```python
from build123d import *

# Parameters (mm, degrees)
F1_DEPTH = 50.8
F2_W     = 22.225
F2_H     = 25.4
F3_DEPTH = 44.704
F4_W     = 22.225
F4_H     = 25.4
F5_DEPTH = 37.592


with BuildPart() as f1:
    # F0 (on Top) → F1 (new body)
    with BuildSketch(Plane.XY):
        Polygon((60.325, 31.75), (-60.325, 31.75), (-60.325, -3.175), (-10.831648, -31.75), (10.831648, -31.75), (60.325, -3.175), align=None)
    extrude(amount=F1_DEPTH)

    # F2 (on Front) → F3 (cut, symmetric)
    with BuildSketch(Plane.XZ):
        with Locations((-49.2125, 38.1)):
            Rectangle(F2_W, F2_H)
    extrude(amount=F3_DEPTH, both=True, mode=Mode.SUBTRACT)

    # F4 (on Front) → F5 (cut, symmetric)
    with BuildSketch(Plane.XZ):
        with Locations((49.2125, 38.1)):
            Rectangle(F4_W, F4_H)
    extrude(amount=F5_DEPTH, both=True, mode=Mode.SUBTRACT)


solid = f1.part
```
The listing builds one solid part. Answer for the finished solid, in the listing's coordinates (mm). A direction names the side the tool comes from. Round coordinates to 2 decimals unless told otherwise and drop trailing zeros. Loops run counter-clockwise (first coordinate to the right, second up) from the corner with the lowest first, then second, coordinate; pieces in that order, holes last. Notation, with made-up numbers: (32, 27.5) -> (68, 27.5) arc R15 cw to (68, 38.5) -> close; hole circle Ø5 at (9.25, -34). An arc over 180 degrees is marked (long way). Use one line per item in the form item = value.
1. A tool of negligible diameter and unlimited length cuts with its end or side. For faces 1 (the flat face through (-38.1, 8, 38)), 2 (the flat face through (60.325, 14, 13)), 3 (the flat face through (38.1, 8, 38)), from which of +Z, -Z, +X, -X, +Y, -Y can it reach the whole face along a straight path? Write none if from no direction.
Answer key:
face_1 = +Z, -X, +Y, -Y
face_2 = +Z, -Z, +X, +Y, -Y
face_3 = +Z, +X, +Y, -Y
2. The part is cut by section D-D on y = -14. Determine the outline of the cut face in (x, z), and give its area (3 significant figures).
Answer key:
outline = (-41.58, 0) -> (41.58, 0) -> (41.58, 25.4) -> (38.1, 25.4) -> (38.1, 50.8) -> (-38.1, 50.8) -> (-38.1, 25.4) -> (-41.58, 25.4) -> close
area = 4,050 mm²
3. The part is cut by section B-B on z = 3. Determine the outline of the cut face in (x, y) (3 decimals), and give its area (3 significant figures).
Answer key:
outline = (-60.325, -3.175) -> (-10.832, -31.75) -> (10.832, -31.75) -> (60.325, -3.175) -> (60.325, 31.75) -> (-60.325, 31.75) -> close
area = 6,250 mm²
4. The part is cut by section A-A on y = 9. Determine the outline of the cut face in (x, z) (3 decimals), and give its area (3 significant figures).
Answer key:
outline = (-60.325, 0) -> (60.325, 0) -> (60.325, 25.4) -> (38.1, 25.4) -> (38.1, 50.8) -> (-38.1, 50.8) -> (-38.1, 25.4) -> (-60.325, 25.4) -> close
area = 5,000 mm²
5. The part is cut by section C-C on x = -51.5. Determine the outline of the cut face in (y, z).
Answer key:
outline = (-8.27, 0) -> (31.75, 0) -> (31.75, 25.4) -> (-8.27, 25.4) -> close
6. Flat-ended cylindrical pins translate along their axes: pin 1 Ø6 at (y, z) = (-14.5, 44) entering from -X; pin 2 Ø7.5 at (y, z) = (19, 34) entering from +X; pin 3 Ø2 at (x, z) = (39.5, 12) entering from -Y; pin 4 Ø24.5 at (x, y) = (50, 18.5) entering from +Z. Find the tip coordinate at first contact, or state that the pin passes through.
Answer key:
pin_1 = -38.1
pin_2 = 38.1
pin_3 = -15.78
pin_4 = 50.8
7. Find the intervals of material crossed by probe 1 along X at (y, z) = (1, 31); probe 2 along Z at (x, y) = (-55, 16.5); probe 3 along Y at (x, z) = (-25.5, 44), in increasing order. Write a range as [from, to].
Answer key:
probe_1 = [-38.1, 38.1]
probe_2 = [0, 25.4]
probe_3 = [-23.28, 31.75]
